For this review, take the finished solid that the model builds, in its own axes (mm). A direction names the side the tool comes from. Give positions to 0.01 mm unless a question says otherwise; leave off trailing zeros. Write each loop counter-clockwise with the first axis right and the second up, starting at its lowest first coordinate (ties: lowest second). Pieces come first, ordered by that corner, then holes. Notation, with made-up numbers: (34.5, 65.25) -> (63.5, 65.25) arc R13 ccw to (63.5, 89.25) -> close; hole circle Ø5 at (42.25, 27). An arc over 180 degrees is marked (long way). Return JSON: item names as keys, results as strings.
from build123d import *

# Parameters (mm, degrees)
SKETCH1_W                      = 30
SKETCH1_H                      = 30
BOSS_EXTRUDE1_DEPTH            = 15
SKETCH2_W                      = 28
SKETCH2_H                      = 28
CUT_EXTRUDE1_DEPTH             = 16
F_3_4_3_4_DIAMETER_HOLE1_D     = 3.4
F_3_4_3_4_DIAMETER_HOLE1_DEPTH = 2
F_3_4_3_4_DIAMETER_HOLE2_D     = 3.4
F_3_4_3_4_DIAMETER_HOLE2_DEPTH = 2
CHAMFER1_SIZE                  = 2
FILLET1_R                      = 1.5875
FILLET2_R                      = 3.5875


with BuildPart() as part:
    # Sketch1 → Boss-Extrude1 (new body)
    with BuildSketch(Plane(origin=(-7.5, 0, 0), x_dir=(0, -1, 0), z_dir=(-1, 0, 0))):
        with Locations((0, 13)):
            Rectangle(SKETCH1_W, SKETCH1_H)
    extrude(amount=-BOSS_EXTRUDE1_DEPTH)

    # Sketch2 → Cut-Extrude1 (cut, through all)
    with BuildSketch(Plane(origin=(7.5, 0, 0), x_dir=(0, 0, -1), z_dir=(1, 0, 0))):
        with Locations((-14, -1)):
            Rectangle(SKETCH2_W, SKETCH2_H)
    extrude(amount=-CUT_EXTRUDE1_DEPTH, mode=Mode.SUBTRACT)

    # Ø3.4 (3.4) Diameter Hole1
    with Locations(Plane.XY):
        with Locations((0, 0), (0, -10)):
            Hole(F_3_4_3_4_DIAMETER_HOLE1_D / 2, depth=F_3_4_3_4_DIAMETER_HOLE1_DEPTH)

    # Ø3.4 (3.4) Diameter Hole2
    with Locations(Plane(origin=(0, 13, 0), x_dir=(-1, 0, 0), z_dir=(0, -1, 0))):
        with Locations((0, -13), (0, -23)):
            Hole(F_3_4_3_4_DIAMETER_HOLE2_D / 2, depth=F_3_4_3_4_DIAMETER_HOLE2_DEPTH)

    # Chamfer1
    chamfer1_edges = [part.edges().sort_by_distance(p)[0] for p in [
        (-7.5, 14, 28),
        (7.5, 14, 28),
        (-7.5, -15, -1),
        (7.5, -15, -1),
    ]]
    chamfer(chamfer1_edges, length=CHAMFER1_SIZE)

    # Fillet1
    fillet1_edges = [part.edges().sort_by_distance(p)[0] for p in [
        (0, 13, 0),
    ]]
    fillet(fillet1_edges, radius=FILLET1_R)

    # Fillet2
    fillet2_edges = [part.edges().sort_by_distance(p)[0] for p in [
        (0, 15, -2),
    ]]
    fillet(fillet2_edges, radius=FILLET2_R)


solid = part.part
1. To check wall thickness, follow probe 1 along X at (y, z) = (13.8, 13); probe 2 along Y at (x, z) = (0, -1.5); probe 3 along Z at (x, y) = (-1.25, 13.25). State the ranges of each line that lie inside material, in increasing order.
Results found:
{"probe 1": "x = -7.5 to -1.7, 1.7 to 7.5", "probe 2": "y = -15 to -11.7, -8.3 to -1.7, 1.7 to 13.24", "probe 3": "z = -1.49 to 11.85, 14.15 to 21.85, 24.15 to 28"}
2. The part is to be moulded in two halves that separate along X. For faces 1 (the cylindrical face through (-0.221, 14.014, 21.314)), 2 (the flat face through (0, 13, 15)), 3 (the flat face through (7.5, 14, 6)), say which applies: +X half, -X half, draft (parallel to the pull), parting line (faces both ways), or undercut.
Results found:
{"face 1": "undercut", "face 2": "draft", "face 3": "+X half"}
3. Add section A-A, the plane z = 13. State the section outline as (x, y) points.
Results found:
{"outline": "(-7.5, 13) -> (-1.7, 13) -> (-1.7, 15) -> (-7.5, 15) -> close; (1.7, 13) -> (7.5, 13) -> (7.5, 15) -> (1.7, 15) -> close"}
4. Add section D-D, the plane x = -6. State the section outline as (y, z) points (1 decimal).
Results found:
{"outline": "(-14.5, -2) -> (11.4, -2) arc R3.6 ccw to (15, 1.6) -> (15, 27.5) -> (13, 27.5) -> (13, 1.6) arc R1.6 cw to (11.4, 0) -> (-14.5, 0) -> close"}
5. Add section B-B, the plane x = 0. State the section outline as (y, z) points (1 decimal), plus the area to 3 significant figures.
Results found:
{"outline": "(-15, -2) -> (-11.7, -2) -> (-11.7, 0) -> (-15, 0) -> close; (-8.3, -2) -> (-1.7, -2) -> (-1.7, 0) -> (-8.3, 0) -> close; (1.7, -2) -> (11.4, -2) arc R3.6 ccw to (15, 1.6) -> (15, 11.3) -> (13, 11.3) -> (13, 1.6) arc R1.6 cw to (11.4, 0) -> (1.7, 0) -> close; (13, 14.7) -> (15, 14.7) -> (15, 21.3) -> (13, 21.3) -> close; (13, 24.7) -> (15, 24.7) -> (15, 28) -> (13, 28) -> close", "area": "86.6 mm²"}
6. For pin 1 (2 mm diameter, centred on x = 2, y = -2.5, fed in from +Z); pin 2 (3 mm diameter, centred on x = 0, z = 13, fed in from +Y); pin 3 (4 mm diameter, centred on x = 0, z = 23, fed in from -Y), all flat-tipped, find the tip position at first contact; note any pin that passes through.
Results found:
{"pin 1": "stops at z = 0", "pin 2": "passes through", "pin 3": "stops at y = 13"}
7. For faces 4 (the flat face through (-6.5, 14, 27)), 5 (the flat face through (0, -2, 0)), list the 3-axis set-ups (+Z, -Z, +X, -X, +Y, -Y) from which the entire face can be reached by the end or side of a thin tool; tool diameter is ignored.
Results found:
{"face 4": "+Z, -X, +Y, -Y", "face 5": "+Z, +X, -X, -Y"}
8. Add section C-C, the plane y = -10. State the section outline as (x, z) points, plus the area to 3 significant figures.
Results found:
{"outline": "(-7.5, -2) -> (-1.7, -2) -> (-1.7, 0) -> (-7.5, 0) -> close; (1.7, -2) -> (7.5, -2) -> (7.5, 0) -> (1.7, 0) -> close", "area": "23.2 mm²"}
